Geometry: final body of the model. Coordinates: model frame, mm. A direction names the side the tool comes from. Round coordinates to 2 decimals unless told otherwise and drop trailing zeros. Order: outer loops, then holes, each group sorted by start corner. A loop starts at its lowest first (then second) coordinate and runs counter-clockwise, first axis right, second up. Notation, with made-up numbers: M 52.5,-18 L 78.5,-18 A31 cw 78.5,17 Z; hole C 80,17.25 d5. An arc over 180 degrees is marked long. Put each result on its own line as item: value. Start each with the question number.
1) Section D-D, the plane y = 0. Count the separate pieces of the cut face and the enclosed holes in it, then the cut area to 3 significant figures.
2) Section B-B, the plane z = 29. Return loops of the section in (x, y).
3) Material intervals for probe 1 along Y at (x, z) = (0, 50); probe 2 along Y at (x, z) = (4.5, 25.5); probe 3 along Z at (x, y) = (14, -24), sorted ascending. Write a range as [from, to].
4) Section C-C, the plane y = -12.5. Return loops of the section in (x, z).
5) Section A-A, the plane x = -18. Return loops of the section in (y, z).
6) Draft query along X for faces 6 (the flat face through (-21.5, -30, 15)), 7 (the flat face through (-27, 16, 55)), 8 (the flat face through (25, -27, 53.22)). Return one class per face: pulls with the +X half, pulls with the -X half, needs draft (parallel to the pull), parting line crosses it, or undercut.
7) Access query for faces 1 (the cylindrical face through (-0.208, 14.086, 1.479)), 2 (the flat face through (24, 17, 26)), 3 (the flat face through (-25, 12.5, 55)), 4 (the cylindrical face through (19.9, -29.48, 13.07)), 5 (the flat face through (-22, 14, 25)). Directions: +Z, -Z, +X, -X, +Y, -Y. A direction counts if a zero-diameter tool reaches every point of the face in a straight line with its end or side. Return the directions, or none.
8) First-contact query: P1, Ø5, axis at y = -24, z = 44, coming from the -X side; P2, Ø3, axis at x = -0.5, y = 14, coming from the +Z side; P3, Ø3, axis at x = 2, y = 0, coming from the -Z side. Flat tips, straight axial feed; report the tip coordinate or a pass-through.
from build123d import *

# Parameters (mm, degrees)
SKETCH_1_W          = 49
SKETCH_1_H          = 51
SKETCH_1_R          = 6
SKETCH_1_R_2        = 1.6
EXTRUDE_1_DEPTH     = 3
SKETCH_2_W          = 49
SKETCH_2_H          = 45
SKETCH_2_W_2        = 16
SKETCH_2_H_2        = 6
EXTRUDE_2_DEPTH     = 3
SKETCH_3_W          = 49
SKETCH_3_H          = 51
SKETCH_3_R          = 1.5
EXTRUDE_3_DEPTH     = 8.22
FILLET_2_R          = 2
FILLET_3_R          = 2
FILLET_4_R          = 2
FILLET_5_R          = 2
FILLET_6_R          = 2
SKETCH_4_W          = 2
SKETCH_4_H          = 3
EXTRUDE_4_DEPTH     = 51
SKETCH_5_W          = 5.5
SKETCH_5_H          = 45.037473363
EXTRUDE_5_DEPTH     = 6
MM_3_D              = 3
MM_3_DEPTH          = 8.22
SKETCH_12_W         = 39.8
SKETCH_12_H         = 4.5
CUT_EXTRUDE_6_DEPTH = 10
SKETCH_13_W         = 2
SKETCH_13_H         = 36
CUT_EXTRUDE_7_DEPTH = 57.22
SKETCH_14_R         = 0.6
CUT_EXTRUDE_8_DEPTH = 52
SKETCH_15_R         = 2
CUT_EXTRUDE_9_DEPTH = 36
SKETCH_16_W         = 38
SKETCH_16_H         = 1.2
EXTRUDE_6_DEPTH     = 35


with BuildPart() as part:
    # 草图1 → 凸台-拉伸1 (new body)
    with BuildSketch(Plane.XY):
        with Locations((-0.5, -5.5)):
            Rectangle(SKETCH_1_W, SKETCH_1_H)
        Circle(SKETCH_1_R, mode=Mode.SUBTRACT)
        with Locations((12.5, 0)):
            Circle(SKETCH_1_R_2, mode=Mode.SUBTRACT)
        with Locations((-12.5, 0)):
            Circle(SKETCH_1_R_2, mode=Mode.SUBTRACT)
        with Locations((0, 12.5)):
            Circle(SKETCH_1_R_2, mode=Mode.SUBTRACT)
        with Locations((0, -12.5)):
            Circle(SKETCH_1_R_2, mode=Mode.SUBTRACT)
    extrude(amount=EXTRUDE_1_DEPTH)

    # 草图2 → 凸台-拉伸2 (add)
    with BuildSketch(Plane.XZ.offset(31)):
        with Locations((-0.5, 25.5)):
            Rectangle(SKETCH_2_W, SKETCH_2_H)
        with Locations((-13.5, 15.5)):
            Rectangle(SKETCH_2_W_2, SKETCH_2_H_2, mode=Mode.SUBTRACT)
        with Locations((12.5, 15.5)):
            Rectangle(SKETCH_2_W_2, SKETCH_2_H_2, mode=Mode.SUBTRACT)
        with Locations((-13.5, 35.5)):
            Rectangle(SKETCH_2_W_2, SKETCH_2_H_2, mode=Mode.SUBTRACT)
        with Locations((12.5, 35.5)):
            Rectangle(SKETCH_2_W_2, SKETCH_2_H_2, mode=Mode.SUBTRACT)
    extrude(amount=-EXTRUDE_2_DEPTH)

    # 草图3 → 凸台-拉伸3 (add)
    with BuildSketch(Plane.XY.offset(48)):
        with Locations((-0.5, -5.5)):
            Rectangle(SKETCH_3_W, SKETCH_3_H)
        with Locations((-12.5, 0)):
            Circle(SKETCH_3_R, mode=Mode.SUBTRACT)
        with Locations((12.5, 0)):
            Circle(SKETCH_3_R, mode=Mode.SUBTRACT)
        with Locations((0, -12.5)):
            Circle(SKETCH_3_R, mode=Mode.SUBTRACT)
        with Locations((0, 12.5)):
            Circle(SKETCH_3_R, mode=Mode.SUBTRACT)
        with Locations((0, 16.75)):
            Circle(SKETCH_3_R, mode=Mode.SUBTRACT)
    extrude(amount=EXTRUDE_3_DEPTH)

    # 圆角2
    fillet_2_edges = [part.edges().sort_by_distance(p)[0] for p in [
        (-5.5, -29.5, 12.5),
    ]]
    fillet(fillet_2_edges, radius=FILLET_2_R)

    # 圆角3
    fillet_3_edges = [part.edges().sort_by_distance(p)[0] for p in [
        (-21.5, -29.5, 12.5),
        (-21.5, -29.5, 18.5),
        (-5.5, -29.5, 18.5),
    ]]
    fillet(fillet_3_edges, radius=FILLET_3_R)

    # 圆角4
    fillet_4_edges = [part.edges().sort_by_distance(p)[0] for p in [
        (20.5, -29.5, 18.5),
        (20.5, -29.5, 12.5),
        (4.5, -29.5, 12.5),
        (4.5, -29.5, 18.5),
        (-21.5, -29.5, 32.5),
        (-21.5, -29.5, 38.5),
        (-5.5, -29.5, 38.5),
        (-5.5, -29.5, 32.5),
        (4.5, -29.5, 32.5),
        (4.5, -29.5, 38.5),
        (20.5, -29.5, 38.5),
        (20.5, -29.5, 32.5),
    ]]
    fillet(fillet_4_edges, radius=FILLET_4_R)

    # 圆角5
    fillet_5_edges = [part.edges().sort_by_distance(p)[0] for p in [
        (-0.5, -28, 3),
    ]]
    fillet(fillet_5_edges, radius=FILLET_5_R)

    # 圆角6
    fillet_6_edges = [part.edges().sort_by_distance(p)[0] for p in [
        (-0.5, -31, 0),
    ]]
    fillet(fillet_6_edges, radius=FILLET_6_R)

    # 草图4 → 凸台-拉伸4 (add)
    with BuildSketch(Plane(origin=(0, -31, 0), x_dir=(-1, 0, 0), z_dir=(0, -1, 0))):
        with Locations((-25, -54.72)):
            Rectangle(SKETCH_4_W, SKETCH_4_H)
        with Locations((26, -54.72)):
            Rectangle(SKETCH_4_W, SKETCH_4_H)
    extrude(amount=-EXTRUDE_4_DEPTH)

    # 草图5 → 凸台-拉伸5 (add)
    with BuildSketch(Plane(origin=(0, 20, 0), x_dir=(1, 0, 0), z_dir=(0, 1, 0))):
        with Locations((-22.25, -25.481263319)):
            Rectangle(SKETCH_5_W, SKETCH_5_H)
        with Locations((21.25, -25.481263319)):
            Rectangle(SKETCH_5_W, SKETCH_5_H)
    extrude(amount=-EXTRUDE_5_DEPTH)

    # 大小mm 暗销孔3
    with Locations(Plane(origin=(0, 0, 48), x_dir=(-1, 0, 0), z_dir=(0, 0, -1))):
        with Locations((15.643749591, 17.172263121), (11.37731054, 17.172263121), (-13.686969003, 17.172263121), (-9.332744424, 17.172263121)):
            Hole(MM_3_D / 2, depth=MM_3_DEPTH)

    # 草图12 → 切除-拉伸6 (cut)
    with BuildSketch(Plane(origin=(0, 20, 0), x_dir=(1, 0, 0), z_dir=(0, 1, 0))):
        with Locations((-0.5, -53.97)):
            Rectangle(SKETCH_12_W, SKETCH_12_H)
    extrude(amount=-CUT_EXTRUDE_6_DEPTH, mode=Mode.SUBTRACT)

    # 草图13 → 切除-拉伸7 (cut, through all)
    with BuildSketch(Plane(origin=(0, 0, 0), x_dir=(-1, 0, 0), z_dir=(0, 0, -1))):
        with Locations((-25, -5.5)):
            Rectangle(SKETCH_13_W, SKETCH_13_H)
        with Locations((26, -5.5)):
            Rectangle(SKETCH_13_W, SKETCH_13_H)
    extrude(amount=-CUT_EXTRUDE_7_DEPTH, mode=Mode.SUBTRACT)

    # 草图14 → 切除-拉伸8 (cut, through all)
    with BuildSketch(Plane(origin=(0, 20, 0), x_dir=(1, 0, 0), z_dir=(0, 1, 0))):
        with Locations((24.9, -54.686530392)):
            Circle(SKETCH_14_R)
        with Locations((-25.9, -54.686530392)):
            Circle(SKETCH_14_R)
    extrude(amount=-CUT_EXTRUDE_8_DEPTH, mode=Mode.SUBTRACT)

    # 草图15 → 切除-拉伸9 (cut)
    with BuildSketch(Plane.XZ.offset(-12.5)):
        with Locations((24.9, 54.686530392)):
            Circle(SKETCH_15_R)
        with Locations((-25.9, 54.686530392)):
            Circle(SKETCH_15_R)
    extrude(amount=CUT_EXTRUDE_9_DEPTH, mode=Mode.SUBTRACT)

    # 草图16 → 凸台-拉伸6 (add)
    with BuildSketch(Plane.XY.offset(3)):
        with Locations((-0.5, 19.4)):
            Rectangle(SKETCH_16_W, SKETCH_16_H)
    extrude(amount=EXTRUDE_6_DEPTH)


solid = part.part
Result sheet:
1. separate pieces: 7
1. enclosed holes: 0
1. area: 440 mm2
2. outline: M -25,-31 L 24,-31 L 24,-28 L -25,-28 Z; M -25,14 L -19.5,14 L -19.5,18.8 L 18.5,18.8 L 18.5,14 L 24,14 L 24,20 L -25,20 Z
3. probe 1: y = [-31, -14], [-11, 11], [14, 15.25], [18.25, 20]
3. probe 2: y = [-31, -28], [18.8, 20]
3. probe 3: z = [0, 3], [48, 56.22]
4. outline: M -25,0 L -1.6,0 L -1.6,3 L -25,3 Z; M -25,48 L -1.5,48 L -1.5,56.22 L -24.62,56.22 A2 cw -25,52.9 Z; M 1.5,48 L 24,48 L 24,52.9 A2 cw 23.62,56.22 L 1.5,56.22 Z; M 1.6,0 L 24,0 L 24,3 L 1.6,3 Z
5. outline: M -31,2 A2 ccw -29,0 L 20,0 L 20,38 L 18.8,38 L 18.8,3 L -26,3 A2 cw -28,5 L -28,12.5 L -31,12.5 Z; M -31,18.5 L -28,18.5 L -28,32.5 L -31,32.5 Z; M -31,38.5 L -28,38.5 L -28,48 L 20,48 L 20,51.72 L 10,51.72 L 10,56.22 L -31,56.22 Z
6. face 6: undercut
6. face 7: pulls with the -X half
6. face 8: needs draft
7. face 1: -Z
7. face 2: -Z, +X, +Y, -Y
7. face 3: -X
7. face 4: -Y
7. face 5: +X, -X
8. P1: passes through
8. P2: stops at z = 51.72
8. P3: stops at z = 48
